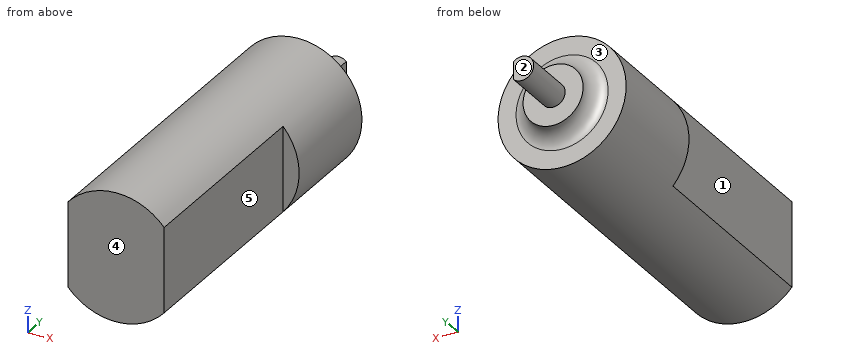
```python
from build123d import *

# Parameters (mm, degrees)
SKETCH1_R           = 8
BOSS_EXTRUDE1_DEPTH = 40.5
SKETCH2_W           = 6
SKETCH2_H           = 10.583005244
CUT_EXTRUDE1_DEPTH  = 26.5
SKETCH3_R           = 3.75
BOSS_EXTRUDE2_DEPTH = 2
FILLET1_R           = 2
SKETCH4_R           = 1.5
BOSS_EXTRUDE3_DEPTH = 7
SKETCH5_W           = 0.5
SKETCH5_H           = 2.236067978
CUT_EXTRUDE2_DEPTH  = 7


with BuildPart() as part:
    # Sketch1 → Boss-Extrude1 (new body)
    with BuildSketch(Plane(origin=(0, 0, 0), x_dir=(1, 0, 0), z_dir=(0, 1, 0))):
        with Locations(Location((0, 0, 0), (0, 0, 270))):
            Circle(SKETCH1_R)
    extrude(amount=BOSS_EXTRUDE1_DEPTH)

    # Sketch2 → Cut-Extrude1 (cut)
    with BuildSketch(Plane(origin=(0, 0, 0), x_dir=(-1, 0, 0), z_dir=(0, -1, 0))):
        with Locations((9, 0)):
            Rectangle(SKETCH2_W, SKETCH2_H)
        with Locations((-9, 0)):
            Rectangle(SKETCH2_W, SKETCH2_H)
    extrude(amount=-CUT_EXTRUDE1_DEPTH, mode=Mode.SUBTRACT)

    # Sketch3 → Boss-Extrude2 (add)
    with BuildSketch(Plane(origin=(0, 40.5, 0), x_dir=(1, 0, 0), z_dir=(0, 1, 0))):
        with Locations(Location((0, 0, 0), (0, 0, 270))):
            Circle(SKETCH3_R)
    extrude(amount=BOSS_EXTRUDE2_DEPTH)

    # Fillet1
    fillet1_edges = [part.edges().sort_by_distance(p)[0] for p in [
        (0, 40.5, -3.75),
    ]]
    fillet(fillet1_edges, radius=FILLET1_R - 0.0001)  # a hair under: the kernel refuses the full size

    # Sketch4 → Boss-Extrude3 (add)
    with BuildSketch(Plane(origin=(0, 42.5, 0), x_dir=(1, 0, 0), z_dir=(0, 1, 0))):
        with Locations(Location((0, 0, 0), (0, 0, 270))):
            Circle(SKETCH4_R)
    extrude(amount=BOSS_EXTRUDE3_DEPTH)

    # Sketch5 → Cut-Extrude2 (cut)
    with BuildSketch(Plane(origin=(0, 49.5, 0), x_dir=(1, 0, 0), z_dir=(0, 1, 0))):
        with Locations((1.25, 0)):
            Rectangle(SKETCH5_W, SKETCH5_H)
    extrude(amount=-CUT_EXTRUDE2_DEPTH, mode=Mode.SUBTRACT)


solid = part.part
```
Design review of the part built by this model. Coordinates are the model's own, in mm. Face numbers are marked on the shaded views. A direction names the side the tool comes from. Give positions to 0.01 mm unless a question says otherwise; leave off trailing zeros. Write each loop counter-clockwise with the first axis right and the second up, starting at its lowest first coordinate (ties: lowest second). Pieces come first, ordered by that corner, then holes.
(1) Clearance check with flat-ended pins moving along their axes: pin 1 Ø5 at (y, z) = (5.5, -4) entering from -X; pin 2 Ø1 at (x, z) = (7, 1) entering from -Y; pin 3 Ø1 at (y, z) = (11, -6.5) entering from +X. State where each tip first meets the part, or that it passes through.
Checked values:
pin 1: stops at x = -6
pin 2: stops at y = 26.5
pin 3: stops at x = 5.29
(2) Wall thickness on line 1 along X through (y, z) = (17, -4.5); line 2 along Y through (x, z) = (-3, 1); line 3 along Y through (x, z) = (-4.25, -3.75): over which ranges is each line inside the solid? List them lowest first.
Checked values:
line 1: x = -6 to 6
line 2: y = 0 to 42.5
line 3: y = 0 to 40.5
(3) Add section D-D (y = 43). Give the boundary of the cut face in (x, z), and give its area (3 significant figures).
Checked values:
outline: (1, -1.12) - (1, 1.12) arc R1.5 ccw (long way) to start
area: 6.29 mm2
(4) Add section C-C (y = 16). Give the boundary of the cut face in (x, z), and give its area (3 significant figures).
Checked values:
outline: (-6, -5.29) arc R8 ccw to (6, -5.29) - (6, 5.29) arc R8 ccw to (-6, 5.29) - close
area: 172 mm2
(5) Tool access review of the marked faces 1, 2, 3, 4 and 5: name each direction out of +Z, -Z, +X, -X, +Y, -Y from which nothing blocks a thin tool from reaching the whole face with its end or side.
Checked values:
face 1: +Z, -Z, -X, -Y
face 2: +Z, -Z, +X, -X, +Y
face 3: +Y
face 4: +Z, -Z, +X, -X, -Y
face 5: +Z, -Z, +X, -Y
